```python
from build123d import *

# Parameters (mm, degrees)
F1_DEPTH    = 5
F2_T1_DEPTH = 18.1085359619
F2_T3_DEPTH = 13.6883237314
F2_T5_DEPTH = 19.2734411819
F2_T7_DEPTH = 13.2933208328


# Not quite as in the source:
# - a fillet or chamfer that OpenCascade refuses, or shapes differently, is made with other operations: its cross-section is extruded or revolved along the edge and cut away or added


with BuildPart() as f1:
    # F0 (on Front) → F1 (new body)
    with BuildSketch(Plane.XZ):
        with BuildLine():
            Line((8.755, -25.285), (8.755, 0))
            ThreePointArc((8.755, 0), (6.0873467679, 6.2923949596), (-0.2899421651, 8.7501976287))
            ThreePointArc((-0.2899421651, 8.7501976287), (-2.9511128894, 8.2426305094), (-5.329706311, 6.9458084942))
            Line((-5.329706311, 6.9458084942), (-3.5034220239, 4.5657484734))
            ThreePointArc((-3.5034220239, 4.5657484734), (5.755, 0), (-3.5034220239, -4.5657484734))
            Line((-3.5034220239, -4.5657484734), (-5.329706311, -6.9458084942))
            ThreePointArc((-5.329706311, -6.9458084942), (-4.2988977903, -7.6268933904), (-3.1824790985, -8.1560929242))
            ThreePointArc((-3.1824790985, -8.1560929242), (-1.3637045363, -8.648140548), (0.5182301058, -8.7396488807))
            ThreePointArc((0.5182301058, -8.7396488807), (3.4984394857, -9.8217007124), (4.755, -12.7326352339))
            Line((4.755, -12.7326352339), (4.755, -14.2977346441))
            ThreePointArc((4.755, -14.2977346441), (3.705175556, -16.9989314509), (1.1067679057, -18.2822370397))
            ThreePointArc((1.1067679057, -18.2822370397), (-0.8255248465, -18.7339906879), (-2.5545928459, -19.7077260178))
            Line((-2.5545928459, -19.7077260178), (-0.7283085589, -22.0877860386))
            ThreePointArc((-0.7283085589, -22.0877860386), (5.755, -25.285), (-0.7283085589, -28.4822139614))
            Line((-0.7283085589, -28.4822139614), (-2.5545928459, -30.8622739822))
            ThreePointArc((-2.5545928459, -30.8622739822), (-0.7476906173, -31.8657827127), (1.2729501298, -32.3004508704))
            ThreePointArc((1.2729501298, -32.3004508704), (6.5334815385, -30.4132945795), (8.755, -25.285))
        make_face()
    extrude(amount=F1_DEPTH)

    # F2: fillet of radius 2 on 8 edges, made by hand

    # F2_s2 → F2_t1 (cut)
    with BuildSketch(Plane.XZ.offset(-6.554267981)):
        with BuildLine():
            ThreePointArc((-3.9278099293, 5.1188215596), (-4.2625544155, 6.8913447905), (-3.0342500285, 8.2123901371))
            ThreePointArc((-3.0342500285, 8.2123901371), (-4.2296570401, 7.6655088757), (-5.329706311, 6.9458084942))
            Line((-5.329706311, 6.9458084942), (-3.9278099293, 5.1188215596))
        make_face()
        with BuildLine():
            ThreePointArc((-3.0342500285, -8.2123901371), (-4.2625544155, -6.8913447905), (-3.9278099293, -5.1188215596))
            Line((-3.9278099293, -5.1188215596), (-5.329706311, -6.9458084942))
            ThreePointArc((-5.329706311, -6.9458084942), (-4.2296570401, -7.6655088757), (-3.0342500285, -8.2123901371))
        make_face()
    extrude(amount=F2_T1_DEPTH, mode=Mode.SUBTRACT)

    # F2_s4 → F2_t3 (cut)
    with BuildSketch(Plane.XZ.offset(-4.3441618657)):
        with BuildLine():
            ThreePointArc((-2.2074106697, 5.3148248452), (-3.4912558515, 5.2297553021), (-4.561245298, 5.9443306041))
            Line((-4.561245298, 5.9443306041), (-3.5034220239, 4.5657484734))
            ThreePointArc((-3.5034220239, 4.5657484734), (-2.8798752345, 4.9826041016), (-2.2074106697, 5.3148248452))
        make_face()
        with BuildLine():
            ThreePointArc((-2.2074106697, -5.3148248452), (-3.4912558515, -5.2297553021), (-4.561245298, -5.9443306041))
            Line((-4.561245298, -5.9443306041), (-3.5034220239, -4.5657484734))
            ThreePointArc((-3.5034220239, -4.5657484734), (-2.8798752345, -4.9826041016), (-2.2074106697, -5.3148248452))
        make_face()
    extrude(amount=F2_T3_DEPTH, mode=Mode.SUBTRACT)

    # F2_s6 → F2_t5 (cut)
    with BuildSketch(Plane.XZ.offset(-7.1367205909)):
        with BuildLine():
            ThreePointArc((0.0158522318, -32.1040698711), (-1.3864892611, -30.8222917209), (-1.084610418, -28.9465555846))
            Line((-1.084610418, -28.9465555846), (-2.5545928459, -30.8622739822))
            ThreePointArc((-2.5545928459, -30.8622739822), (-1.3330660217, -31.6150183417), (0.0158522318, -32.1040698711))
        make_face()
        with BuildLine():
            ThreePointArc((-1.084610418, -21.6234444154), (-1.3864892611, -19.7477082791), (0.0158522318, -18.4659301289))
            ThreePointArc((0.0158522318, -18.4659301289), (-1.3330660217, -18.9549816583), (-2.5545928459, -19.7077260178))
            Line((-2.5545928459, -19.7077260178), (-1.084610418, -21.6234444154))
        make_face()
    extrude(amount=F2_T5_DEPTH, mode=Mode.SUBTRACT)

    # F2_s8 → F2_t7 (cut)
    with BuildSketch(Plane.XZ.offset(-4.1466604164)):
        with BuildLine():
            ThreePointArc((0.4709999062, -21.4550673942), (-0.7422563844, -21.46506549), (-1.7380393272, -20.7718792817))
            Line((-1.7380393272, -20.7718792817), (-0.7283085589, -22.0877860386))
            ThreePointArc((-0.7283085589, -22.0877860386), (-0.1554567483, -21.7206231375), (0.4709999062, -21.4550673942))
        make_face()
        with BuildLine():
            ThreePointArc((-1.7380393272, -29.7981207183), (-0.7422563844, -29.10493451), (0.4709999062, -29.1149326058))
            ThreePointArc((0.4709999062, -29.1149326058), (-0.1554567483, -28.8493768625), (-0.7283085589, -28.4822139614))
            Line((-0.7283085589, -28.4822139614), (-1.7380393272, -29.7981207183))
        make_face()
    extrude(amount=F2_T7_DEPTH, mode=Mode.SUBTRACT)


solid = f1.part
```
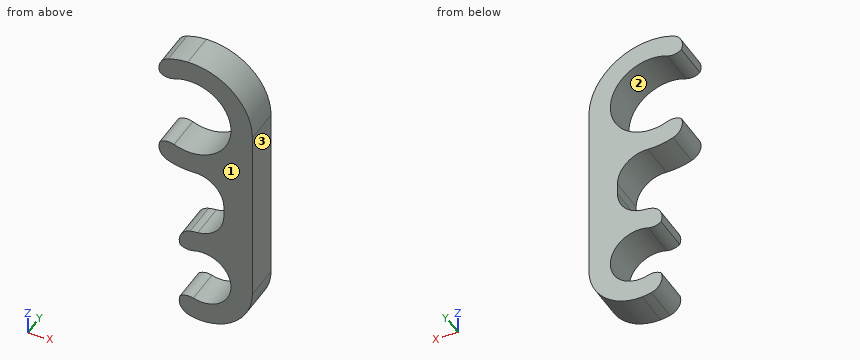
Work out the finished part from the listing and answer in its coordinate system (mm). Face numbers are marked on the shaded views. Give positions to 0.01 mm unless a question says otherwise; leave off trailing zeros. Loops run counter-clockwise (first coordinate to the right, second up) from the corner with the lowest first, then second, coordinate; pieces in that order, holes last. Notation, with made-up numbers: (61.25, 1) -> (79.25, 1) arc R14 ccw to (79.25, 17) -> close; hole circle Ø10 at (29.5, -27). An arc over 180 degrees is marked (long way). Use CSV: the item, a comma, the result in double quotes.
1. Straight lines are drawn through the part: line 1 (Z direction, x = 0, y = -3.7) (3 decimals); line 2 (Z direction, x = 0.25, y = -1.3); line 3 (X direction, y = -2, z = -12.5) (3 decimals). For each, find the intervals that lie inside material, in ascending order.
Found:
line 1,"-32.1 to -29.021, -21.549 to -18.47, -8.755 to -5.755, 5.755 to 8.755"
line 2,"-32.16 to -29.06, -21.51 to -18.41, -8.75 to -5.75, 5.75 to 8.75"
line 3,"4.748 to 8.755"
2. The part is cut by section B-B (x = 5.25). Write down the section's boundary in (y, z), then the cut area to 3 significant figures.
Found:
outline,"(-5, -31.37) -> (0, -31.37) -> (0, -27.24) -> (-5, -27.24) -> close; (-5, -23.33) -> (0, -23.33) -> (0, -2.36) -> (-5, -2.36) -> close; (-5, 2.36) -> (0, 2.36) -> (0, 7.01) -> (-5, 7.01) -> close"
area,"149 mm^2"
3. The mould has two halves that part along X. Classify the marked faces 1, 2 and 3: +X half, -X half, draft (parallel to the pull), parting line (faces both ways), or undercut.
Found:
face 1,"draft"
face 2,"undercut"
face 3,"+X half"
4. The part is cut by section C-C (y = -4.55). Write down the section's boundary in (x, z) (1 decimal), then the cut area to 3 significant figures.
Found:
outline,"(-4.2, -5.6) arc R2 ccw to (-3, -8.2) arc R8.8 ccw to (0.5, -8.7) arc R4 cw to (4.8, -12.7) -> (4.8, -14.3) arc R4 cw to (1.1, -18.3) arc R7 ccw to (0, -18.5) arc R2 ccw to (-1.4, -21.2) arc R2 ccw to (0.5, -21.5) arc R4 cw (long way) to (0.5, -29.1) arc R2 ccw to (-1.4, -29.4) arc R2 ccw to (0, -32.1) arc R7 ccw to (8.8, -25.3) -> (8.8, 0) arc R8.8 ccw to (-3, 8.2) arc R2 ccw to (-4.2, 5.6) arc R2 ccw to (-2.2, 5.3) arc R5.8 cw (long way) to (-2.2, -5.3) arc R2 ccw to start"
area,"235 mm^2"
5. Flat-ended cylindrical pins translate along their axes: pin 1 Ø1.5 at (x, y) = (7.5, -3.5) entering from -Z; pin 2 Ø1.7 at (y, z) = (-3.5, -13) entering from -X. Find the tip coordinate at first contact, or state that the pin passes through.
Found:
pin 1,"z = -30.2"
pin 2,"x = 4.71"
6. The part is cut by section A-A (x = 3.5). Write down the section's boundary in (y, z), then the cut area to 3 significant figures.
Found:
outline,"(-5, -32.09) -> (0, -32.09) -> (0, -28.9) -> (-5, -28.9) -> close; (-5, -21.67) -> (0, -21.67) -> (0, -17.21) -> (-5, -17.21) -> close; (-5, -9.82) -> (0, -9.82) -> (0, -4.57) -> (-5, -4.57) -> close; (-5, 4.57) -> (0, 4.57) -> (0, 8.02) -> (-5, 8.02) -> close"
area,"81.8 mm^2"
7. The part is cut by section D-D (z = -26.5). Write down the section's boundary in (x, y).
Found:
outline,"(5.57, -5) -> (8.65, -5) -> (8.65, 0) -> (5.57, 0) -> close"
